Print and shaded views of the part. All mm, measured from the part's lowest x, y and z. Coordinates: 2 decimals unless noted, no trailing zeros. Order: outer loops, then holes, each group sorted by start corner. A loop starts at its lowest first (then second) coordinate and runs counter-clockwise, first axis right, second up. Notation, with made-up numbers: (-27.5, -9) -> (7.5, -9) arc R33 ccw to (7.5, 20) -> close; hole circle Ø3 at (76, 60). An arc over 180 degrees is marked (long way). Return JSON: item names as keys, results as strings. Group by question number.
1) Probe line 1 (X direction, y = 76, z = 0.45); line 2 (Y direction, x = 81, z = 1.65); line 3 (Y direction, x = 101.35, z = 0.85). List the from-to ranges inside material, lowest first.
2) Cut at B-B (y = 70). Write the cut outline in (x, z).
3) Cut at D-D (x = 31). Write the cut outline in (y, z).
4) Cut at C-C (y = 30.5). Write the cut outline in (x, z).
5) Flat gauge pins, fed straight in: pin 1 (3 mm diameter, centred on x = 31, y = 80.5, fed in from +Z); pin 2 (1 mm diameter, centred on y = 3, z = 0.5, fed in from -X). Where does each tip first touch, or does it go through?
6) Cut at A-A (x = 74.5). Write the cut outline in (y, z).
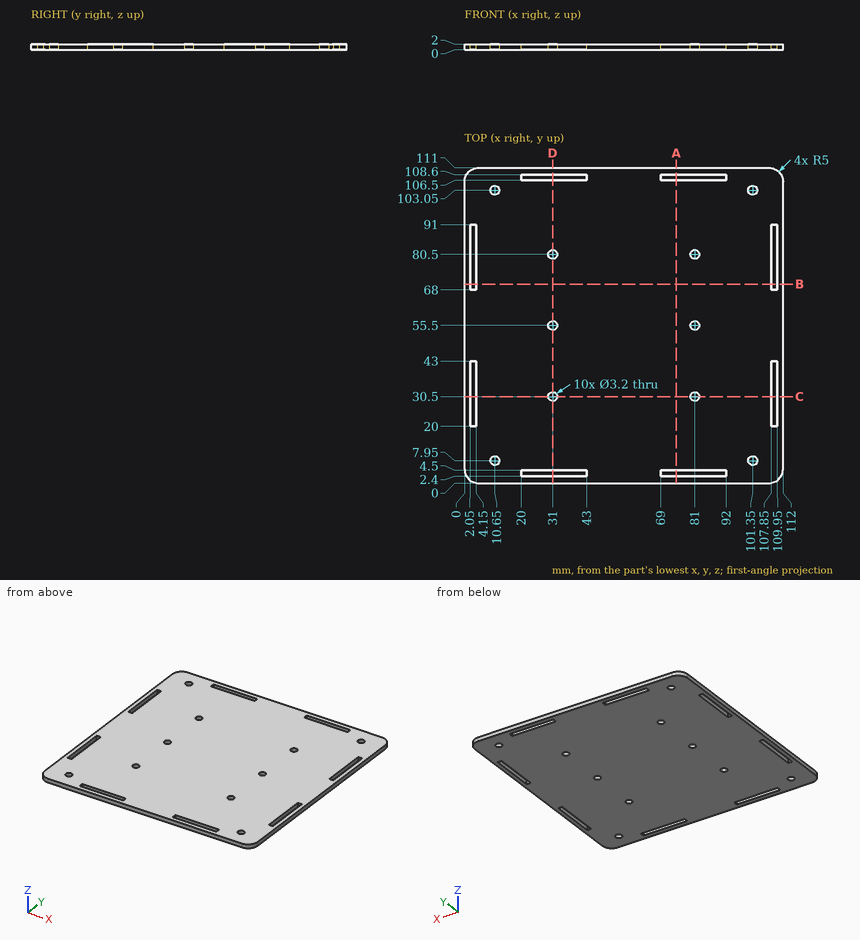
Answers below:
{
 "1": {"line 1": "x = 0 to 2.05, 4.15 to 107.85, 109.95 to 112", "line 2": "y = 0 to 2.4, 4.5 to 28.9, 32.1 to 53.9, 57.1 to 78.9, 82.1 to 106.5, 108.6 to 111", "line 3": "y = 0 to 6.35, 9.55 to 101.45, 104.65 to 111"},
 "2": {"outline": "(0, 0) -> (2.05, 0) -> (2.05, 2) -> (0, 2) -> close; (4.15, 0) -> (107.85, 0) -> (107.85, 2) -> (4.15, 2) -> close; (109.95, 0) -> (112, 0) -> (112, 2) -> (109.95, 2) -> close"},
 "3": {"outline": "(0, 0) -> (2.4, 0) -> (2.4, 2) -> (0, 2) -> close; (4.5, 0) -> (28.9, 0) -> (28.9, 2) -> (4.5, 2) -> close; (32.1, 0) -> (53.9, 0) -> (53.9, 2) -> (32.1, 2) -> close; (57.1, 0) -> (78.9, 0) -> (78.9, 2) -> (57.1, 2) -> close; (82.1, 0) -> (106.5, 0) -> (106.5, 2) -> (82.1, 2) -> close; (108.6, 0) -> (111, 0) -> (111, 2) -> (108.6, 2) -> close"},
 "4": {"outline": "(0, 0) -> (2.05, 0) -> (2.05, 2) -> (0, 2) -> close; (4.15, 0) -> (29.4, 0) -> (29.4, 2) -> (4.15, 2) -> close; (32.6, 0) -> (79.4, 0) -> (79.4, 2) -> (32.6, 2) -> close; (82.6, 0) -> (107.85, 0) -> (107.85, 2) -> (82.6, 2) -> close; (109.95, 0) -> (112, 0) -> (112, 2) -> (109.95, 2) -> close"},
 "5": {"pin 1": "passes through", "pin 2": "stops at x = 0.23"},
 "6": {"outline": "(0, 0) -> (2.4, 0) -> (2.4, 2) -> (0, 2) -> close; (4.5, 0) -> (106.5, 0) -> (106.5, 2) -> (4.5, 2) -> close; (108.6, 0) -> (111, 0) -> (111, 2) -> (108.6, 2) -> close"}
}
